```python
from build123d import *

# Parameters (mm, degrees)
F1_DEPTH = 20
F2_DEPTH = 50
F3_DEPTH = 30


with BuildPart() as f1:
    # F0 (on Top) → F1 (new body)
    with BuildSketch(Plane.XY):
        Polygon((-20.765196, 62.555887), (-2.182231, 30.369248), (4.086395, 30.369248), (-16.063726, 65.270282), align=None)
        Polygon((-27.913605, 30.369248), (-27.913605, 23.369248), (-3.063605, 23.369248), (-2.913605, 23.369248), (-2.913605, 4.369248), (-3.063605, 4.369248), (-13.063605, 4.369248), (-13.063605, -2.630752), (4.086395, -2.630752), (4.086395, 30.369248), (-2.182231, 30.369248), align=None)
        Polygon((20.252203, 2.369248), (4.086395, 30.369248), (4.086395, -2.630752), (23.138954, -2.630752), align=None)
        Polygon((28.912457, 7.369248), (20.252203, 2.369248), (23.138954, -2.630752), (31.799208, 2.369248), align=None)
        Polygon((26.96224, 10.861619), (28.912457, 7.369248), (31.799208, 2.369248), (35.26331, 4.369248), (30.376763, 12.832995), align=None)
    extrude(amount=F1_DEPTH)

    # F0 (on Top) → F2 (join)
    with BuildSketch(Plane.XY):
        Polygon((-20.765196, 62.555887), (-2.182231, 30.369248), (4.086395, 30.369248), (-16.063726, 65.270282), align=None)
        Polygon((-27.913605, 30.369248), (-27.913605, 23.369248), (-3.063605, 23.369248), (-2.913605, 23.369248), (-2.913605, 4.369248), (-3.063605, 4.369248), (-13.063605, 4.369248), (-13.063605, -2.630752), (4.086395, -2.630752), (4.086395, 30.369248), (-2.182231, 30.369248), align=None)
        Polygon((20.252203, 2.369248), (4.086395, 30.369248), (4.086395, -2.630752), (23.138954, -2.630752), align=None)
        Polygon((28.912457, 7.369248), (20.252203, 2.369248), (23.138954, -2.630752), (31.799208, 2.369248), align=None)
        Polygon((26.96224, 10.861619), (28.912457, 7.369248), (31.799208, 2.369248), (35.26331, 4.369248), (30.376763, 12.832995), align=None)
    extrude(amount=-F2_DEPTH)

    # F0 (on Top) → F3 (cut)
    with BuildSketch(Plane.XY):
        Polygon((-20.765196, 62.555887), (-2.182231, 30.369248), (4.086395, 30.369248), (-16.063726, 65.270282), align=None)
        Polygon((28.912457, 7.369248), (20.252203, 2.369248), (23.138954, -2.630752), (31.799208, 2.369248), align=None)
        Polygon((26.96224, 10.861619), (28.912457, 7.369248), (31.799208, 2.369248), (35.26331, 4.369248), (30.376763, 12.832995), align=None)
    extrude(amount=-F3_DEPTH, mode=Mode.SUBTRACT)


solid = f1.part
```
Verification items for the finished model (mm, model axes). A direction names the side the tool comes from. Coordinates: 2 decimals unless noted, no trailing zeros. Write each loop counter-clockwise with the first axis right and the second up, starting at its lowest first coordinate (ties: lowest second). Pieces come first, ordered by that corner, then holes. Notation, with made-up numbers: M 14.5,86 L 64.5,86 A15 ccw 64.5,101 Z; hole C 41.5,88.25 d1. An arc over 180 degrees is marked long. One line per item, written item: value.
Item 1: Section check A-A, the plane x = -17. Record the boundary of the cut face in (y, z), plus the area to 3 significant figures.
Check sheet entries:
outline: M 23.37,-50 L 30.37,-50 L 30.37,20 L 23.37,20 Z; M 56.03,-50 L 64.73,-50 L 64.73,-30 L 56.03,-30 Z; M 56.03,0 L 64.73,0 L 64.73,20 L 56.03,20 Z
area: 838 mm^2
Item 2: Section check C-C, the plane y = 38. Record the boundary of the cut face in (x, z), plus the area to 3 significant figures.
Check sheet entries:
outline: M -6.59,-50 L -0.32,-50 L -0.32,-30 L -6.59,-30 Z; M -6.59,0 L -0.32,0 L -0.32,20 L -6.59,20 Z
area: 251 mm^2
Item 3: Mould release check, pull along Z, two halves, no side actions. Record for faces 1 (the flat face through (-8, 47, 0)), 2 (the flat face through (32.854, 8.542, -39.86)), 3 (the flat face through (1, 19, 20)): pulls with the +Z half, pulls with the -Z half, needs draft (parallel to the pull), parting line crosses it, or undercut.
Check sheet entries:
face 1: undercut
face 2: needs draft
face 3: pulls with the +Z half
Item 4: Access from +Z, -Z, +X, -X, +Y, -Y to the whole of each face (thin tool, end or side, straight path). Record for faces 4 (the flat face through (28, 9, 10)), 5 (the flat face through (-2.914, 14, -15)), 6 (the flat face through (-8, 47, -30)), 7 (the flat face through (28.69, 11.86, 10.14)).
Check sheet entries:
face 4: +Z, -Z
face 5: +Z, -Z, -X
face 6: +X, -X, +Y
face 7: +Z, -Z, +Y
Item 5: Section check B-B, the plane z = 11. Record the boundary of the cut face in (x, y), plus the area to 3 significant figures.
Check sheet entries:
outline: M -27.91,23.37 L -2.91,23.37 L -2.91,4.37 L -13.06,4.37 L -13.06,-2.63 L 23.14,-2.63 L 35.26,4.37 L 30.38,12.83 L 26.96,10.86 L 28.91,7.37 L 20.25,2.37 L -16.06,65.27 L -20.77,62.56 L -2.18,30.37 L -27.91,30.37 Z
area: 1,100 mm^2
Item 6: Scan lines: line 1 along Y through (x, z) = (-15.5, -18); line 2 along Z through (x, y) = (-10.5, 50); line 3 along Y through (x, z) = (-11.5, -13). Record each from-to range of solid material in increasing order.
Check sheet entries:
line 1: y = 23.37 to 30.37
line 2: z = -50 to -30, 0 to 20
line 3: y = -2.63 to 4.37, 23.37 to 30.37
Item 7: Gauge pin test, flat ends, axial feed: pin 1 Ø1.5 at (y, z) = (38.5, -40) entering from -X; pin 2 Ø12.5 at (x, y) = (-2.5, 53.5) entering from +Z; pin 3 Ø10 at (y, z) = (16, -26.5) entering from +X; pin 4 Ø5 at (x, z) = (0.5, -19.5) entering from +Y. Record the tip position at first contact, or that the pin passes through.
Check sheet entries:
pin 1: stops at x = -7.31
pin 2: stops at z = 20
pin 3: stops at x = 30.61
pin 4: stops at y = 30.37
Item 8: Section check D-D, the plane x = 1.5. Record the boundary of the cut face in (y, z).
Check sheet entries:
outline: M -2.63,-50 L 34.85,-50 L 34.85,-30 L 30.37,-30 L 30.37,0 L 34.85,0 L 34.85,20 L -2.63,20 Z
